Part model, mm, in its own coordinate system. A direction names the side the tool comes from. Give positions to 0.01 mm unless a question says otherwise; leave off trailing zeros. Order: outer loops, then holes, each group sorted by start corner. A loop starts at its lowest first (then second) coordinate and runs counter-clockwise, first axis right, second up.
1. Slice it at A-A on x = -7.5. List the corners of the cut face in (y, z), and give its area (3 significant figures).
2. Drop a flat-ended pin along its axis: pin 1 Ø1 at (x, y) = (-27.5, 6) entering from +Z. Give the stop position or say it passes through.
3. Which spindle directions (+Z, -Z, +X, -X, +Y, -Y) get a long thin tool onto all of the face, cutting with end or side? Do faces 5 (the flat face through (0, 5, -15)), 6 (the cylindrical face through (-37.297, 5.07, -13.986)). Say none if no direction does.
4. Slice it at B-B on y = 8.25. Give the number of separate pieces and of enclosed holes in the cut face, and give its area (3 significant figures).
5. Probe line 1 (Z direction, x = -16, y = 9.75); line 2 (X direction, y = 6.25, z = 8); line 3 (X direction, y = 2.25, z = 7.5). List the from-to ranges inside material, lowest first.
6. Mould opens along X. For faces 1 (the flat face through (-1, 0, 18)), 2 (the flat face through (25, 5, 0)), 3 (the cylindrical face through (-29.165, 4.93, 1.562)), 4 (the cylindrical face through (-37.297, 5.07, 13.986)) say: +X half, -X half, draft (parallel to the pull), parting line (faces both ways), or undercut.
7. Slice it at C-C on z = 9.5. List the corners of the cut face in (x, y), and give its area (3 significant figures).
from build123d import *

# Parameters (mm, degrees)
F0_W     = 86
F0_H     = 40
F1_DEPTH = 10
F2_R     = 5.2
F3_DEPTH = 25
F4_W     = 50
F4_H     = 30
F5_DEPTH = 25
F6_R     = 19.99999


# Not quite as in the source:
# - a fillet or chamfer is up to 0.001 mm smaller than in the source, because OpenCascade refuses the exact size


with BuildPart() as f1:
    # F0 (on Front) → F1 (new body)
    with BuildSketch(Plane.XZ):
        Rectangle(F0_W, F0_H)
    extrude(amount=-F1_DEPTH)

    # F2 (on face) → F3 (cut)
    with BuildSketch(Plane.XZ):
        with Locations((-34.125, 0)):
            Circle(F2_R)
        with Locations((34.125, 0)):
            Circle(F2_R)
    extrude(amount=-F3_DEPTH, mode=Mode.SUBTRACT)

    # F4 (on face) → F5 (cut)
    with BuildSketch(Plane.XZ):
        Rectangle(F4_W, F4_H)
    extrude(amount=-F5_DEPTH, mode=Mode.SUBTRACT)

    # F6 (radius 20 in the source; OpenCascade refuses exactly that, so slightly less here)
    f6_edges = [f1.edges().sort_by_distance(p)[0] for p in [
        (-43, 5, 20),
        (43, 5, 20),
        (43, 5, -20),
        (-43, 5, -20),
    ]]
    fillet(f6_edges, radius=F6_R)


solid = f1.part
Data:
1. outline: (0, -20) - (10, -20) - (10, -15) - (0, -15) - close; (0, 15) - (10, 15) - (10, 20) - (0, 20) - close
1. area: 100 mm2
2. pin 1: stops at z = 19.6
3. face 5: +Y, -Y
3. face 6: -Z, -X, +Y, -Y
4. separate pieces: 1
4. enclosed holes: 3
4. area: 1,430 mm2
5. line 1: z = -20 to -15, 15 to 20
5. line 2: x = -41.33 to -25, 25 to 41.33
5. line 3: x = -41.54 to -25, 25 to 41.54
6. face 1: draft
6. face 2: undercut
6. face 3: undercut
6. face 4: -X half
7. outline: (-40.6, 0) - (-25, 0) - (-25, 10) - (-40.6, 10) - close; (25, 0) - (40.6, 0) - (40.6, 10) - (25, 10) - close
7. area: 312 mm2
